from build123d import *

# Parameters (mm, degrees)
SKETCH1_R            = 190.5
BOSS_EXTRUDE1_DEPTH  = 57.15
SKETCH2_R            = 19.05
CUT_EXTRUDE1_DEPTH   = 484.378
SKETCH3_R            = 127
CUT_EXTRUDE2_DEPTH   = 6.35
SKETCH4_R            = 63.5
CUT_EXTRUDE3_DEPTH   = 19.05
FILLET1_R            = 20.32
FILLET2_R            = 20.32
FILLET3_R            = 30.48
FILLET4_R            = 30.48
FILLET1_OF_MIRROR2_R = 20.32
FILLET2_OF_MIRROR2_R = 20.32
FILLET3_OF_MIRROR2_R = 30.48
FILLET4_OF_MIRROR2_R = 30.48
FILLET7_R            = 25.4
FILLET8_R            = 25.4
SKETCH5_R            = 51.013146757
BOSS_EXTRUDE3_DEPTH  = 76.2
SKETCH6_R            = 12.7
CUT_EXTRUDE4_DEPTH   = 1040.638


with BuildPart() as part:
    # Sketch1 → Boss-Extrude1 (new body)
    with BuildSketch(Plane(origin=(0, 0, 0), x_dir=(1, 0, 0), z_dir=(0, 1, 0))):
        with Locations(Location((0, 0, 0), (0, 0, 270))):
            Circle(SKETCH1_R)
    boss_extrude1 = extrude(amount=BOSS_EXTRUDE1_DEPTH)

    # Sketch2 → Cut-Extrude1 (cut)
    with BuildSketch(Plane(origin=(0, 57.15, 0), x_dir=(1, 0, 0), z_dir=(0, 1, 0))):
        with Locations(Location((0, 0, 0), (0, 0, 270))):
            Circle(SKETCH2_R)
    cut_extrude1 = extrude(amount=-CUT_EXTRUDE1_DEPTH, mode=Mode.SUBTRACT)

    # Sketch3 → Cut-Extrude2 (cut)
    with BuildSketch(Plane(origin=(0, 0, 0), x_dir=(-1, 0, 0), z_dir=(0, -1, 0))):
        with Locations(Location((0, 0, 0), (0, 0, 90))):
            Circle(SKETCH3_R)
    cut_extrude2 = extrude(amount=-CUT_EXTRUDE2_DEPTH, mode=Mode.SUBTRACT)

    # Sketch4 → Cut-Extrude3 (cut)
    with BuildSketch(Plane(origin=(0, 0, 0), x_dir=(1, 0, 0), z_dir=(0, 1, 0))):
        with Locations(Location((0, 0, 0), (0, 0, 90))):
            Circle(SKETCH4_R)
    cut_extrude3 = extrude(amount=CUT_EXTRUDE3_DEPTH, mode=Mode.SUBTRACT)

    # Fillet1
    # the kernel refuses this fillet: 20.32 mm, written as the material it takes off along each edge
    with BuildSketch(Plane(origin=(0, 0, 0), x_dir=(0, 0, -1), z_dir=(-1, 0, 0))) as fillet1_piece_1:
        with BuildLine():
            CenterArc((141.756066549, -20.32), FILLET1_R, 90, 46.567463442)
            Line((127, -6.35), (126.704878669, -6.0706))
            ThreePointArc((126.704878669, -6.0706), (126.5936, -3.175), (126.5936, 0))
            Line((126.5936, 0), (127, 0.4064))
            Line((127, 0.4064), (141.756066549, 0.4064))
            Line((141.756066549, 0.4064), (141.756066549, 0))
        make_face()
    revolve(axis=Axis((0, 0, 0), (0, -1, 0)), mode=Mode.SUBTRACT)

    # Fillet2
    fillet2_edges = [part.edges().sort_by_distance(p)[0] for p in [
        (0, 6.35, 127),
    ]]
    fillet(fillet2_edges, radius=FILLET2_R)

    # Fillet3
    # the kernel refuses this fillet: 30.48 mm, written as the material it takes off along each edge
    with BuildSketch(Plane(origin=(0, 6.35, 0), x_dir=(0, 0, -1), z_dir=(-1, 0, 0))) as fillet3_piece_1:
        with BuildLine():
            CenterArc((88.256857636, -30.48), FILLET3_R, 90, 54.314665287)
            Line((63.5, -12.7), (63.004862847, -12.3444))
            ThreePointArc((63.004862847, -12.3444), (62.8904, -6.35), (62.8904, 0))
            Line((62.8904, 0), (63.5, 0.6096))
            Line((63.5, 0.6096), (88.256857636, 0.6096))
            Line((88.256857636, 0.6096), (88.256857636, 0))
        make_face()
    revolve(axis=Axis((0, 6.35, 0), (0, -1, 0)), mode=Mode.SUBTRACT)

    # Fillet4
    fillet4_edges = [part.edges().sort_by_distance(p)[0] for p in [
        (0, 19.05, 63.5),
    ]]
    fillet(fillet4_edges, radius=FILLET4_R)

    # Mirror2: Boss-Extrude1, Cut-Extrude1, Cut-Extrude2, Cut-Extrude3 across plane
    add(boss_extrude1.mirror(Plane.ZX.offset(57.15)))
    add(cut_extrude1.mirror(Plane.ZX.offset(57.15)), mode=Mode.SUBTRACT)
    add(cut_extrude2.mirror(Plane.ZX.offset(57.15)), mode=Mode.SUBTRACT)
    add(cut_extrude3.mirror(Plane.ZX.offset(57.15)), mode=Mode.SUBTRACT)

    # Fillet1 of Mirror2
    # the kernel refuses this fillet: 20.32 mm, written as the material it takes off along each edge
    with BuildSketch(Plane(origin=(0, 114.3, 0), x_dir=(0, 0, -1), z_dir=(-1, 0, 0))) as fillet1_of_mirror2_piece_1:
        with BuildLine():
            CenterArc((141.756066549, 20.32), FILLET1_OF_MIRROR2_R, 223.432536558, 46.567463442)
            Line((127, 6.35), (126.704878669, 6.0706))
            ThreePointArc((126.704878669, 6.0706), (126.5936, 3.175), (126.5936, 0))
            Line((126.5936, 0), (127, -0.4064))
            Line((127, -0.4064), (141.756066549, -0.4064))
            Line((141.756066549, -0.4064), (141.756066549, 0))
        make_face()
    revolve(axis=Axis((0, 114.3, 0), (0, -1, 0)), mode=Mode.SUBTRACT)

    # Fillet2 of Mirror2
    fillet2_of_mirror2_edges = [part.edges().sort_by_distance(p)[0] for p in [
        (0, 107.95, 127),
    ]]
    fillet(fillet2_of_mirror2_edges, radius=FILLET2_OF_MIRROR2_R)

    # Fillet3 of Mirror2
    # the kernel refuses this fillet: 30.48 mm, written as the material it takes off along each edge
    with BuildSketch(Plane(origin=(0, 107.95, 0), x_dir=(0, 0, -1), z_dir=(1, 0, 0))) as fillet3_of_mirror2_piece_1:
        with BuildLine():
            CenterArc((88.256857636, -30.48), FILLET3_OF_MIRROR2_R, 90, 54.314665287)
            Line((63.5, -12.7), (63.004862847, -12.3444))
            ThreePointArc((63.004862847, -12.3444), (62.8904, -6.35), (62.8904, 0))
            Line((62.8904, 0), (63.5, 0.6096))
            Line((63.5, 0.6096), (88.256857636, 0.6096))
            Line((88.256857636, 0.6096), (88.256857636, 0))
        make_face()
    revolve(axis=Axis((0, 107.95, 0), (0, 1, 0)), mode=Mode.SUBTRACT)

    # Fillet4 of Mirror2
    fillet4_of_mirror2_edges = [part.edges().sort_by_distance(p)[0] for p in [
        (0, 95.25, 63.5),
    ]]
    fillet(fillet4_of_mirror2_edges, radius=FILLET4_OF_MIRROR2_R)

    # Fillet7
    fillet7_edges = [part.edges().sort_by_distance(p)[0] for p in [
        (0, 114.3, -190.5),
    ]]
    fillet(fillet7_edges, radius=FILLET7_R)

    # Fillet8
    fillet8_edges = [part.edges().sort_by_distance(p)[0] for p in [
        (0, 0, -190.5),
    ]]
    fillet(fillet8_edges, radius=FILLET8_R)

    # Sketch5 → Boss-Extrude3 (add)
    with BuildSketch(Plane(origin=(0, 95.25, 0), x_dir=(1, 0, 0), z_dir=(0, 1, 0))):
        Circle(SKETCH5_R)
    extrude(amount=-BOSS_EXTRUDE3_DEPTH)

    # Sketch6 → Cut-Extrude4 (cut)
    with BuildSketch(Plane(origin=(0, 95.25, 0), x_dir=(1, 0, 0), z_dir=(0, 1, 0))):
        with Locations(Location((0, 0, 0), (0, 0, 270))):
            Circle(SKETCH6_R)
    extrude(amount=-CUT_EXTRUDE4_DEPTH, mode=Mode.SUBTRACT)


solid = part.part
The model under review builds one solid part; all positions refer to its coordinate system, in mm. A direction names the side the tool comes from. Round coordinates to 2 decimals unless told otherwise and drop trailing zeros. Loops run counter-clockwise (first coordinate to the right, second up) from the corner with the lowest first, then second, coordinate; pieces in that order, holes last. Notation, with made-up numbers: (36, -17) -> (66, -17) arc R7 ccw to (66, -12) -> close; hole circle Ø5 at (75, 38.5). An arc over 180 degrees is marked (long way). Write item = value, one per line. Start each with the question number.
Item 1: Take a section at A-A on y = 79.5. Give the boundary of the cut face in (x, z).
Item 2: To check wall thickness, follow L1, parallel to X at y = 54, z = 0; L2, parallel to Y at x = 83.5, z = -88; L3, parallel to Y at x = 83, z = -59.5. State the ranges of each line that lie inside material, in increasing order.
Item 3: Mouldability with a two-part tool opening along X and no side actions: class faces 4 (the flat face through (70, 107.95, 54)), 5 (the cylindrical face through (-185.97, 56.71, -41.3)), 6 (the flat face through (123, 0, 73)) as released by +X, released by -X, zero draft, split by the parting line, or undercut.
Item 4: For faces 1 (the flat face through (12, 19.05, -11)), 2 (the flat face through (123, 114.3, 73)), 3 (the flat face through (12, 95.25, -11)), list the 3-axis set-ups (+Z, -Z, +X, -X, +Y, -Y) from which the entire face can be reached by the end or side of a thin tool; tool diameter is ignored.
Item 5: Insertion check: pin 1 (1 mm diameter, centred on x = 113.5, z = -5.5, fed in from +Y); pin 2 (2 mm diameter, centred on x = -82, z = -5.5, fed in from -Y); pin 3 (1.5 mm diameter, centred on y = 75, z = -32, fed in from +X). Each pin has a flat end and moves straight along its axis. Give the tip position at first contact, or say it passes through.
Result:
q1.outline = circle Ø381 at (0, 0); hole circle Ø25.4 at (0, 0)
q2.L1 = -190.5 to -12.7, 12.7 to 190.5
q2.L2 = 6.3 to 108
q2.L3 = 6.35 to 107.95
q3.face_4 = undercut
q3.face_5 = split by the parting line
q3.face_6 = zero draft
q4.face_1 = -Y
q4.face_2 = +Z, -Z, +X, -X, +Y
q4.face_3 = +Y
q5.pin_1 = 107.95
q5.pin_2 = 6.78
q5.pin_3 = 187.92
